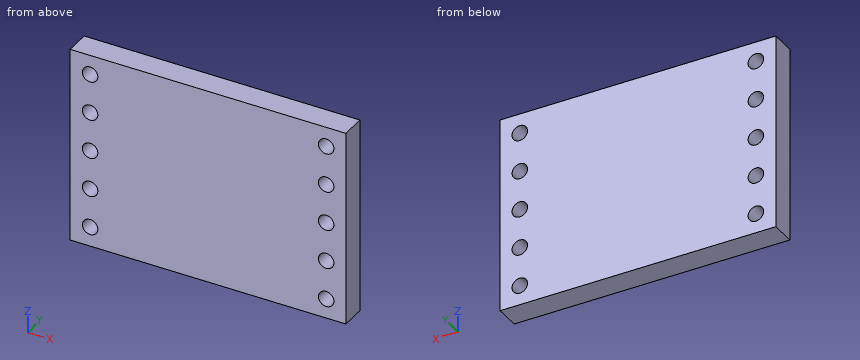
Autodesk Inventor part; units mm, degrees
ref_plane "Work Plane1" through (0, 8.55, 0) normal (0, 1, 0) x (1, 0, 0)
ref_plane "Work Plane2" through (0, -20.05, 0) normal (0, -1, 0) x (1, 0, 0)
ref_plane "YZ Plane" through (0, 0, 0) normal (1, 0, 0) x (0, 1, 0)
sketch "Sketch2" plane through (0, 0, 0) normal (0, 1, 0) x (-1, 0, 0)
  line L0 (-8.9, 6.35) -> (8.9, 6.35)
  line L1 (8.9, 6.35) -> (8.9, -6.35)
  line L2 (8.9, -6.35) -> (-8.9, -6.35)
  line L3 (-8.9, -6.35) -> (-8.9, 6.35)
  line L4 (-8.9, 6.35) -> (8.9, -6.35) construction
  line L5 (8.9, 6.35) -> (-8.9, -6.35) construction
  circle A0 centre (-7.63, 5.08) radius 0.5
  circle A1 centre (-7.63, 2.54) radius 0.5
  circle A2 centre (-7.63, -2.54) radius 0.5
  circle A3 centre (-7.63, -5.08) radius 0.5
  circle A4 centre (7.61, -5.08) radius 0.5
  circle A5 centre (7.61, -2.54) radius 0.5
  circle A6 centre (7.61, 0) radius 0.5
  circle A7 centre (7.61, 2.54) radius 0.5
  circle A8 centre (7.61, 5.08) radius 0.5
  circle A9 centre (-7.63, 0) radius 0.5
  point P0 (0, 0)
  point P1 (-7.63, -5.08)
  point P2 (-7.63, -2.54)
  point P3 (-7.63, 0)
  point P4 (-7.63, 2.54)
  point P5 (7.61, -2.54)
  point P6 (7.61, 2.54)
  dimension "d1" = 17.8
  dimension "d2" = 12.7
  dimension "d5" = 1.27
  dimension "d6" = 1.27
  dimension "d9" = 2.54
  dimension "d12" = 15.24
  dimension "d15" = 1
  dimension "d20" = 1
  dimension "d25" = 1
  dimension "d30" = 1
  dimension "d35" = 1
  dimension "d40" = 1
  dimension "d45" = 1
  dimension "d50" = 1
  dimension "d55" = 1
  dimension "d60" = 1
extrude "Extrusion2" add sketch "Sketch2" along normal mid plane 1.6
ref_plane "Work Plane1" through (0, 8.55, 0) normal (0, 1, 0) x (1, 0, 0)
sketch "Sketch3" plane through (0, 8.55, 0) normal (0, 1, 0) x (1, 0, 0)
  line L0 (-8.9372, -7.2611) -> (-8.9372, 7.6441) construction
  line L1 (-8.9372, 7.6441) -> (9.9152, 7.6441) construction
  line L2 (9.9152, 7.6441) -> (9.9152, -7.2611) construction
  line L3 (9.9152, -7.2611) -> (-8.9372, -7.2611) construction
  circle A0 centre (7.63, 0) radius 0.5
  circle A1 centre (-7.61, -5.08) radius 0.5
  circle A2 centre (-7.61, -2.54) radius 0.5
  circle A3 centre (-7.61, 0) radius 0.5
  circle A4 centre (-7.61, 2.54) radius 0.5
  circle A5 centre (-7.61, 5.08) radius 0.5
  circle A6 centre (7.63, 5.08) radius 0.5
  circle A7 centre (7.63, 2.54) radius 0.5
  circle A8 centre (7.63, -2.54) radius 0.5
  circle A9 centre (7.63, -5.08) radius 0.5
  line L4 (-8.9, -6.35) -> (8.9, -6.35)
  line L5 (8.9, -6.35) -> (8.9, 6.35)
  line L6 (8.9, 6.35) -> (-8.9, 6.35)
  line L7 (-8.9, 6.35) -> (-8.9, -6.35)
  point P0 (0, 0)
decal "Decal1"
ref_plane "Work Plane2" through (0, -20.05, 0) normal (0, -1, 0) x (1, 0, 0)
sketch "Sketch4" plane through (0, -20.05, 0) normal (0, -1, 0) x (1, 0, 0)
  line L0 (-9.0888, -7.7888) -> (-9.0888, 7.0827) construction
  line L1 (-9.0888, 7.0827) -> (9.7209, 7.0827) construction
  line L2 (9.7209, 7.0827) -> (9.7209, -7.7888) construction
  line L3 (9.7209, -7.7888) -> (-9.0888, -7.7888) construction
  circle A0 centre (7.63, 0) radius 0.5
  circle A1 centre (-7.61, 5.08) radius 0.5
  circle A2 centre (-7.61, 2.54) radius 0.5
  circle A3 centre (-7.61, 0) radius 0.5
  circle A4 centre (-7.61, -2.54) radius 0.5
  circle A5 centre (-7.61, -5.08) radius 0.5
  circle A6 centre (7.63, -5.08) radius 0.5
  circle A7 centre (7.63, -2.54) radius 0.5
  circle A8 centre (7.63, 2.54) radius 0.5
  circle A9 centre (7.63, 5.08) radius 0.5
  line L4 (8.9, 6.35) -> (-8.9, 6.35)
  line L5 (-8.9, 6.35) -> (-8.9, -6.35)
  line L6 (-8.9, -6.35) -> (8.9, -6.35)
  line L7 (8.9, -6.35) -> (8.9, 6.35)
  point P0 (0, 0)
decal "Decal2"
properties part number "microsdadapterboard" material "GFRC"
Source: CAD feature listing. Evaluate the final solid. Frame: model axes, mm. Round coordinates to 2 decimals unless told otherwise and drop trailing zeros. Loops run counter-clockwise (first coordinate to the right, second up) from the corner with the lowest first, then second, coordinate; pieces in that order, holes last.
Q1. Section B-B, the plane z = 5.08. Return loops of the section in (x, y), plus the area to 3 significant figures.
Q2. Ray query, line 1 (Z direction, x = -7.61, y = -0.1); line 2 (X direction, y = 0.75, z = 4.75); line 3 (X direction, y = -0.1, z = -5.25). Return the intervals inside material, ascending.
Q3. Section A-A, the plane x = 7.63. Return loops of the section in (y, z), plus the area to 3 significant figures.
Q4. Section C-C, the plane y = -0.25. State how many separate pieces and enclosed holes the cut face has, plus the area to 3 significant figures.
Q5. Section D-D, the plane z = -2.75. Return loops of the section in (x, y).
Solutions:
1. outline: (-8.9, -0.8) - (-8.11, -0.8) - (-8.11, 0.8) - (-8.9, 0.8) - close; (-7.11, -0.8) - (7.13, -0.8) - (7.13, 0.8) - (-7.11, 0.8) - close; (8.13, -0.8) - (8.9, -0.8) - (8.9, 0.8) - (8.13, 0.8) - close
1. area: 25.3 mm2
2. line 1: z = -6.35 to -5.58, -4.58 to -3.04, -2.04 to -0.5, 0.5 to 2.04, 3.04 to 4.58, 5.58 to 6.35
2. line 2: x = -8.9 to -7.99, -7.23 to 7.25, 8.01 to 8.9
2. line 3: x = -8.9 to -8.08, -7.14 to 7.16, 8.1 to 8.9
3. outline: (-0.8, -6.35) - (0.8, -6.35) - (0.8, -5.58) - (-0.8, -5.58) - close; (-0.8, -4.58) - (0.8, -4.58) - (0.8, -3.04) - (-0.8, -3.04) - close; (-0.8, -2.04) - (0.8, -2.04) - (0.8, -0.5) - (-0.8, -0.5) - close; (-0.8, 0.5) - (0.8, 0.5) - (0.8, 2.04) - (-0.8, 2.04) - close; (-0.8, 3.04) - (0.8, 3.04) - (0.8, 4.58) - (-0.8, 4.58) - close; (-0.8, 5.58) - (0.8, 5.58) - (0.8, 6.35) - (-0.8, 6.35) - close
3. area: 12.3 mm2
4. separate pieces: 1
4. enclosed holes: 10
4. area: 218 mm2
5. outline: (-8.9, -0.8) - (-8.06, -0.8) - (-8.06, 0.8) - (-8.9, 0.8) - close; (-7.16, -0.8) - (7.18, -0.8) - (7.18, 0.8) - (-7.16, 0.8) - close; (8.08, -0.8) - (8.9, -0.8) - (8.9, 0.8) - (8.08, 0.8) - close
